```python
from build123d import *

# Parameters (mm, degrees)
SKETCH_1_W          = 166.48
SKETCH_1_H          = 51.75
EXTRUDE_1_DEPTH     = 3
SKETCH_3_R          = 1.6
CUT_EXTRUDE_2_DEPTH = 10
SKETCH_4_R          = 1.6
CUT_EXTRUDE_3_DEPTH = 10


with BuildPart() as part:
    # 草图1 → 凸台-拉伸1 (new body)
    with BuildSketch(Plane(origin=(0, 0, 0), x_dir=(1, 0, 0), z_dir=(0, 1, 0))):
        with Locations((0, 25.875)):
            Rectangle(SKETCH_1_W, SKETCH_1_H)
    extrude(amount=EXTRUDE_1_DEPTH)

    # 草图3 → 切除-拉伸2 (cut)
    with BuildSketch(Plane(origin=(0, 3, 0), x_dir=(1, 0, 0), z_dir=(0, 1, 0))):
        with Locations(Location((-18, 44.25, 0), (0, 0, 270))):
            Circle(SKETCH_3_R)
        with Locations(Location((0, 42.25, 0), (0, 0, 270))):
            Circle(SKETCH_3_R)
        with Locations(Location((18, 44.25, 0), (0, 0, 270))):
            Circle(SKETCH_3_R)
    extrude(amount=-CUT_EXTRUDE_2_DEPTH, mode=Mode.SUBTRACT)

    # 草图4 → 切除-拉伸3 (cut)
    with BuildSketch(Plane(origin=(0, 3, 0), x_dir=(1, 0, 0), z_dir=(0, 1, 0))):
        with Locations(Location((0, 10.65378949, 0), (0, 0, 270))):
            Circle(SKETCH_4_R)
        with Locations(Location((18, 8.65378949, 0), (0, 0, 270))):
            Circle(SKETCH_4_R)
        with Locations(Location((-18, 7.5, 0), (0, 0, 270))):
            Circle(SKETCH_4_R)
    extrude(amount=-CUT_EXTRUDE_3_DEPTH, mode=Mode.SUBTRACT)


solid = part.part
```
The model under review builds one solid part; all positions refer to its coordinate system, in mm. Coordinates: 2 decimals unless noted, no trailing zeros. Write each loop counter-clockwise with the first axis right and the second up, starting at its lowest first coordinate (ties: lowest second). Pieces come first, ordered by that corner, then holes. Notation, with made-up numbers: (55, 43) - (99, 43) arc R25 cw to (99, 71) - close; hole circle Ø11 at (69, 74.25). An arc over 180 degrees is marked (long way). Answer in a Markdown table with one row per item. Add a question column.
Q1. Consider section A-A on x = 0. Give the boundary of the cut face in (y, z), then the cut area to 3 significant figures.
Q2. To check wall thickness, follow line 1 along X through (y, z) = (2.1, -44.25); line 2 along X through (y, z) = (1.3, -42); line 3 along Z through (x, y) = (1, 2.2). State the ranges of each line that lie inside material, in increasing order. Write a range as from..to.
Q3. Draft analysis for pull direction Z (two halves, no side actions). For faces 1 (the face through (-1, 1, -51.75)), 2 (the face through (-83.24, 1, -26)), 3 (the face through (0.07, 1.521, -12.252)), state which applies: +Z half, -Z half, draft (parallel to the pull), parting line (faces both ways), or undercut.
Answers below:
| question | item | result |
|---|---|---|
| 1 | outline | (0, -51.75) - (3, -51.75) - (3, -43.85) - (0, -43.85) - close; (0, -40.65) - (3, -40.65) - (3, -12.25) - (0, -12.25) - close; (0, -9.05) - (3, -9.05) - (3, 0) - (0, 0) - close |
| 1 | area | 136 mm² |
| 2 | line 1 | -83.24..-19.6, -16.4..16.4, 19.6..83.24 |
| 2 | line 2 | -83.24..-1.58, 1.58..83.24 |
| 2 | line 3 | -51.75..-43.5, -41..-11.9, -9.4..0 |
| 3 | face 1 | -Z half |
| 3 | face 2 | draft |
| 3 | face 3 | undercut |
